Verification items for the finished model (mm, model axes). A direction names the side the tool comes from. Coordinates: 2 decimals unless noted, no trailing zeros. Order: outer loops, then holes, each group sorted by start corner. A loop starts at its lowest first (then second) coordinate and runs counter-clockwise, first axis right, second up. Notation, with made-up numbers: (22.25, 6.5) -> (70.25, 6.5) arc R15 ccw to (70.25, 15.5) -> close; hole circle Ø9 at (81.5, 31.25). An arc over 180 degrees is marked (long way). Write each question's results on one line, items separated by ' | '. Start each with the question number.
(1) Cross-section at B-B on z = 19. Enter the section's corners in (x, y).
(2) Thickness scan on probe 1 along Y at (x, z) = (19, 7); probe 2 along X at (y, z) = (-18.05, -8.5); probe 3 along Z at (x, y) = (15, 0.25). Record the ranges inside material, lowest first. Write a range as [from, to].
(3) Go/stop test with flat-tipped pins: pin 1 (8 mm diameter, centred on x = -3, y = -9.5, fed in from -Z); pin 2 (1 mm diameter, centred on x = 12, y = -6.5, fed in from -Z); pin 3 (5 mm diameter, centred on x = -1.48, z = -16.94, fed in from -Y) (3 decimals); pin 4 (3 mm diameter, centred on x = 3, y = -18.5, fed in from -Z). Record where each tip stops, or that it passes through.
(4) Cross-section at D-D on y = -2.75. Enter the section's corners in (x, z), and give its area (3 significant figures).
(5) Set-up check for faces 5 (the cylindrical face through (17.45, 1.48, -8.86)), 6 (the flat face through (-20.32, -17.48, 5.33)), 7 (the flat face through (13, -16, -10)), 8 (the flat face through (20.32, -17.48, -5.33)), 9 (the cylindrical face through (-6.834, -7.888, -1.517)): record each of +Z, -Z, +X, -X, +Y, -Y from which the full face is reachable in a straight line by a thin tool's end or side.
(6) Cross-section at C-C on x = 5. Enter the section's corners in (y, z), and give its area (3 significant figures).
(7) Cross-section at A-A on z = 0. Enter the section's corners in (x, y).
(8) Draft check along Y on faces 1 (the cylindrical face through (-11.42, -7.89, 8.36)), 2 (the flat face through (-7.3, -19.5, 0)), 3 (the cylindrical face through (9.991, -7.888, -7.883)), 4 (the flat face through (-4, 3, 0)). Enter one of: +Y half, -Y half, draft (parallel to the pull), parting line (faces both ways), or undercut.
```python
from build123d import *

# Parameters (mm, degrees)
SKETCH1_R           = 7
SKETCH1_R_2         = 2.75
BOSS_EXTRUDE1_DEPTH = 3
SKETCH2_R           = 7
BOSS_EXTRUDE2_DEPTH = 16
SKETCH3_R           = 7
BOSS_EXTRUDE3_DEPTH = 26
CUT_EXTRUDE1_DEPTH  = 9
SKETCH5_R           = 9
SKETCH5_R_2         = 7
BOSS_EXTRUDE4_DEPTH = 0.5
SKETCH6_R           = 2.5
CUT_EXTRUDE2_DEPTH  = 17


with BuildPart() as part:
    # Sketch1 → Boss-Extrude1 (new body)
    with BuildSketch(Plane(origin=(0, 0, 0), x_dir=(1, 0, 0), z_dir=(0, 1, 0))):
        with BuildLine():
            Line((19.48717527, -4.5), (21.126127543, -6.138952274))
            ThreePointArc((21.126127543, -6.138952274), (0, -22), (-21.126127543, -6.138952274))
            Line((-21.126127543, -6.138952274), (-19.48717527, -4.5))
            ThreePointArc((-19.48717527, -4.5), (-20, 0), (-19.48717527, 4.5))
            Line((-19.48717527, 4.5), (-21.126127543, 6.138952274))
            ThreePointArc((-21.126127543, 6.138952274), (0, 22), (21.126127543, 6.138952274))
            Line((21.126127543, 6.138952274), (19.48717527, 4.5))
            ThreePointArc((19.48717527, 4.5), (20, 0), (19.48717527, -4.5))
        make_face()
        with Locations(Location((0, 0, 0), (0, 0, 270))):
            Circle(SKETCH1_R, mode=Mode.SUBTRACT)
        with Locations(Location((0, -17, 0), (0, 0, 270))):
            Circle(SKETCH1_R_2, mode=Mode.SUBTRACT)
        with Locations(Location((-14.722431864, 8.5, 0), (0, 0, 270))):
            Circle(SKETCH1_R_2, mode=Mode.SUBTRACT)
        with Locations(Location((14.722431864, 8.5, 0), (0, 0, 270))):
            Circle(SKETCH1_R_2, mode=Mode.SUBTRACT)
        with Locations(Location((15.40723238, -7.18451045, 0), (0, 0, 270))):
            Circle(SKETCH1_R_2, mode=Mode.SUBTRACT)
        with Locations(Location((-13.925584753, -9.750799418, 0), (0, 0, 270))):
            Circle(SKETCH1_R_2, mode=Mode.SUBTRACT)
        with Locations(Location((-1.481647627, 16.935309868, 0), (0, 0, 270))):
            Circle(SKETCH1_R_2, mode=Mode.SUBTRACT)
    boss_extrude1 = extrude(amount=BOSS_EXTRUDE1_DEPTH)

    # Sketch2 → Boss-Extrude2 (add)
    with BuildSketch(Plane.XZ):
        with Locations(Location((-8.5, 14.722431864, 0), (0, 0, 67.839045349))):
            Circle(SKETCH2_R)
        with Locations(Location((8.5, -14.722431864, 0), (0, 0, 60.223318028))):
            Circle(SKETCH2_R)
    extrude(amount=BOSS_EXTRUDE2_DEPTH)

    # Mirror1: Boss-Extrude1 across plane
    add(boss_extrude1.mirror(Plane(origin=(0, -8, 0), x_dir=(0, 0, 1), z_dir=(0, -1, 0))))

    # Sketch3 → Boss-Extrude3 (add)
    with BuildSketch(Plane(origin=(0, 3, 0), x_dir=(1, 0, 0), z_dir=(0, 1, 0))):
        with Locations(Location((0, 0, 0), (0, 0, 270))):
            Circle(SKETCH3_R)
    extrude(amount=-BOSS_EXTRUDE3_DEPTH)

    # Sketch4 → Cut-Extrude1 (cut)
    with BuildSketch(Plane.XZ.offset(23)):
        with BuildLine():
            Line((1, -1), (1, -3.872983346))
            ThreePointArc((1, -3.872983346), (0, -4), (-1, -3.872983346))
            Line((-1, -3.872983346), (-1, -1))
            Line((-1, -1), (-3.872983346, -1))
            ThreePointArc((-3.872983346, -1), (-4, 0), (-3.872983346, 1))
            Line((-3.872983346, 1), (-1, 1))
            Line((-1, 1), (-1, 3.872983346))
            ThreePointArc((-1, 3.872983346), (0, 4), (1, 3.872983346))
            Line((1, 3.872983346), (1, 1))
            Line((1, 1), (3.872983346, 1))
            ThreePointArc((3.872983346, 1), (4, 0), (3.872983346, -1))
            Line((3.872983346, -1), (1, -1))
        make_face()
    extrude(amount=-CUT_EXTRUDE1_DEPTH, mode=Mode.SUBTRACT)

    # Sketch5 → Boss-Extrude4 (add)
    with BuildSketch(Plane.XZ.offset(19)):
        with Locations(Location((0, 0, 0), (0, 0, 270))):
            Circle(SKETCH5_R)
        with Locations(Location((0, 0, 0), (0, 0, 90))):
            Circle(SKETCH5_R_2, mode=Mode.SUBTRACT)
    extrude(amount=BOSS_EXTRUDE4_DEPTH)

    # Sketch6 → Cut-Extrude2 (cut)
    with BuildSketch(Plane(origin=(0, 3, 0), x_dir=(1, 0, 0), z_dir=(0, 1, 0))):
        with Locations(Location((0, 0, 0), (0, 0, 270))):
            Circle(SKETCH6_R)
    extrude(amount=-CUT_EXTRUDE2_DEPTH, mode=Mode.SUBTRACT)


solid = part.part
```
Results are:
1) outline: (-14.04, -16) -> (-11.09, -16) -> (-11.09, -19) -> (-1.89, -19) -> (-1.89, -16) -> (-2.96, -16) -> (-2.96, 0) -> (-1.89, 0) -> (-1.89, 3) -> (-11.09, 3) -> (-11.09, 0) -> (-14.04, 0) -> close; (1.89, -19) -> (11.09, -19) -> (11.09, -16) -> (1.89, -16) -> close; (1.89, 0) -> (11.09, 0) -> (11.09, 3) -> (1.89, 3) -> close
2) probe 1: y = [-19, -16], [0, 3] | probe 2: x = [-20.29, -17.47], [-11.97, 11.97], [17.47, 20.29] | probe 3: z = [-16.09, -11.24], [-5.76, 4.46], [9.9, 16.09]
3) pin 1: stops at z = -7 | pin 2: stops at z = -21.05 | pin 3: passes through | pin 4: stops at z = -21.95
4) outline: circle Ø14 at (-8.5, 14.72); circle Ø14 at (0, 0); circle Ø14 at (8.5, -14.72); hole circle Ø5 at (0, 0) | area: 442 mm2
5) face 5: +Y | face 6: -X, +Y, -Y | face 7: -Y | face 8: +X, +Y, -Y | face 9: none
6) outline: (-23, -4.9) -> (-19.5, -4.9) -> (-19.5, -7.48) -> (-19, -7.48) -> (-19, -21.42) -> (-16, -21.42) -> (-16, -20.78) -> (0, -20.78) -> (0, -21.42) -> (3, -21.42) -> (3, 21.42) -> (0, 21.42) -> (0, 4.9) -> (-16, 4.9) -> (-16, 21.42) -> (-19, 21.42) -> (-19, 7.48) -> (-19.5, 7.48) -> (-19.5, 4.9) -> (-23, 4.9) -> close; hole (-16, -8.66) -> (0, -8.66) -> (0, -4.9) -> (-16, -4.9) -> close | area: 650 mm2
7) outline: (-20, -19) -> (-9, -19) -> (-9, -19.5) -> (-7, -19.5) -> (-7, -23) -> (-4, -23) -> (-4, -14) -> (-2.5, -14) -> (-2.5, 3) -> (-20, 3) -> (-20, 0) -> (-7, 0) -> (-7, -16) -> (-20, -16) -> close; (2.5, -14) -> (4, -14) -> (4, -23) -> (7, -23) -> (7, -19.5) -> (9, -19.5) -> (9, -19) -> (20, -19) -> (20, -16) -> (7, -16) -> (7, 0) -> (20, 0) -> (20, 3) -> (2.5, 3) -> close
8) face 1: undercut | face 2: -Y half | face 3: undercut | face 4: +Y half
